from build123d import *

# Parameters (mm, degrees)
BOSS_EXTRUDE1_DEPTH = 3.175


with BuildPart() as part:
    # Sketch1 → Boss-Extrude1 (new body)
    with BuildSketch(Plane(origin=(0, 0, 0), x_dir=(1, 0, 0), z_dir=(0, 1, 0))):
        with BuildLine():
            Line((0, 29.6545), (0, 6.35))
            ThreePointArc((0, 6.35), (-6.35, 0), (0, -6.35))
            Line((0, -6.35), (0, -29.6545))
            ThreePointArc((0, -29.6545), (29.6545, 0), (0, 29.6545))
        make_face()
        with BuildLine():
            Line((6.35, 22.422694313), (6.35, 3.666174209))
            Line((6.35, 3.666174209), (20.182289022, 11.65225))
            ThreePointArc((20.182289022, 11.65225), (14.317514025, 18.387727222), (6.35, 22.422694313))
        make_face(mode=Mode.SUBTRACT)
        with BuildLine():
            Line((6.35, 0), (21.581607168, -8.793972499))
            ThreePointArc((21.581607168, -8.793972499), (23.3045, 0), (21.581607168, 8.793972499))
            Line((21.581607168, 8.793972499), (6.35, 0))
        make_face(mode=Mode.SUBTRACT)
        with BuildLine():
            Line((6.35, -3.666174209), (20.182289022, -11.65225))
            ThreePointArc((20.182289022, -11.65225), (14.317514025, -18.387727222), (6.35, -22.422694313))
            Line((6.35, -22.422694313), (6.35, -3.666174209))
        make_face(mode=Mode.SUBTRACT)
    extrude(amount=BOSS_EXTRUDE1_DEPTH)


solid = part.part
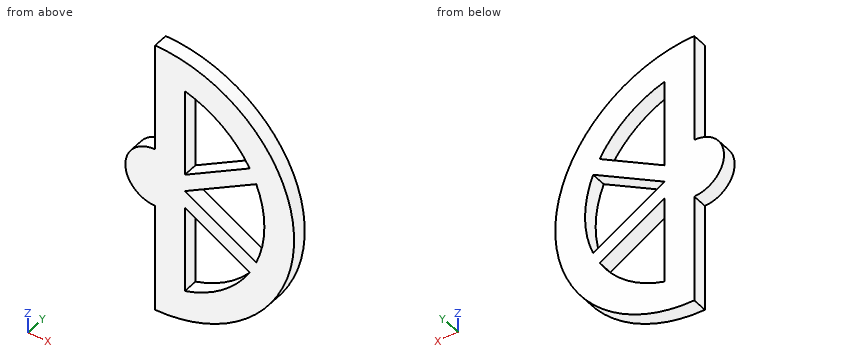
Check sheet for the modelled part. Datum: model origin and axes. Units: mm. Round coordinates to 2 decimals unless told otherwise and drop trailing zeros. Loops run counter-clockwise (first coordinate to the right, second up) from the corner with the lowest first, then second, coordinate; pieces in that order, holes last.
1. Sectioned sample at B-B on x = 13. Record the boundary of the cut face in (y, z) (3 decimals).
2. Sectioned sample at C-C on z = 20. Record the boundary of the cut face in (x, y) (3 decimals), and give its area (3 significant figures).
3. Sectioned sample at A-A on y = 2.6. Record the boundary of the cut face in (x, z), and give its area (3 significant figures).
4. Gauge pin test, flat ends, axial feed: pin 1 Ø1 at (y, z) = (2, -22.5) entering from -X; pin 2 Ø1 at (x, y) = (6, 1) entering from +Z. Record the tip position at first contact, or that the pin passes through.
5. Scan lines: probe 1 along Z at (x, y) = (17, 1.6); probe 2 along Z at (x, y) = (14, 0.65); probe 3 along X at (y, z) = (2.1, 14). Record each from-to range of solid material in increasing order.
Recorded:
1. outline: (0, -26.653) - (3.175, -26.653) - (3.175, -19.342) - (0, -19.342) - close; (0, -7.506) - (3.175, -7.506) - (3.175, -3.839) - (0, -3.839) - close; (0, 3.839) - (3.175, 3.839) - (3.175, 7.506) - (0, 7.506) - close; (0, 19.342) - (3.175, 19.342) - (3.175, 26.653) - (0, 26.653) - close
2. outline: (0, 0) - (6.35, 0) - (6.35, 3.175) - (0, 3.175) - close; (11.962, 0) - (21.895, 0) - (21.895, 3.175) - (11.962, 3.175) - close
2. area: 51.7 mm2
3. outline: (0, -29.65) arc R29.65 ccw to (0, 29.65) - (0, 6.35) arc R6.35 ccw to (0, -6.35) - close; hole (6.35, -22.42) arc R23.3 ccw to (20.18, -11.65) - (6.35, -3.67) - close; hole (6.35, 0) - (21.58, -8.79) arc R23.3 ccw to (21.58, 8.79) - close; hole (6.35, 3.67) - (20.18, 11.65) arc R23.3 ccw to (6.35, 22.42) - close
3. area: 991 mm2
4. pin 1: stops at x = 0
4. pin 2: stops at z = 29.14
5. probe 1: z = -24.3 to -15.94, -9.81 to -6.15, 6.15 to 9.81, 15.94 to 24.3
5. probe 2: z = -26.14 to -18.63, -8.08 to -4.42, 4.42 to 8.08, 18.63 to 26.14
5. probe 3: x = 0 to 6.35, 18.63 to 26.14
